Geometry: final body of the model. Coordinates: model frame, mm. Give positions to 0.01 mm unless a question says otherwise; leave off trailing zeros. Loops run counter-clockwise (first coordinate to the right, second up) from the corner with the lowest first, then second, coordinate; pieces in that order, holes last.
Autodesk Inventor part; units mm, degrees
ref_plane "YZ Plane" through (0, 0, 0) normal (1, 0, 0) x (0, 1, 0)
ref_plane "XZ Plane" through (0, 0, 0) normal (0, 1, 0) x (-1, 0, 0)
ref_plane "XY Plane" through (0, 0, 0) normal (0, 0, 1) x (1, 0, 0)
sketch "Sketch2" plane through (0, 0, 0) normal (1, 0, 0) x (0, 1, 0)
  line L0 (0, -180) -> (0, 0)
  line L1 (0, 0) -> (30, 0)
  line L2 (30, 0) -> (30, -3)
  line L3 (30, -3) -> (60, -3)
  line L4 (60, -3) -> (60, 0)
  line L5 (60, 0) -> (90, 0)
  line L6 (90, 0) -> (90, -3)
  line L7 (90, -3) -> (120, -3)
  line L8 (120, -3) -> (120, 0)
  line L9 (120, 0) -> (150, 0)
  line L10 (150, 0) -> (150, -3)
  line L11 (150, -3) -> (180, -3)
  line L12 (180, -3) -> (180, 0)
  line L13 (180, 0) -> (210, 0)
  line L14 (210, 0) -> (210, -3)
  line L15 (210, -3) -> (240, -3)
  line L16 (240, -3) -> (240, 0)
  line L17 (240, 0) -> (250, 0)
  line L18 (153.75, -180) -> (153.75, -80)
  line L19 (153.75, -80) -> (250, 0)
  line L20 (0, -90) -> (37, -90) construction
  line L21 (0, -180) -> (30, -180)
  line L22 (30, -180) -> (30, -177)
  line L23 (30, -177) -> (60, -177)
  line L24 (60, -177) -> (60, -180)
  line L25 (60, -180) -> (90, -180)
  line L26 (90, -180) -> (90, -177)
  line L27 (90, -177) -> (120, -177)
  line L28 (120, -177) -> (120, -180)
  line L29 (120, -180) -> (150, -180)
  line L30 (150, -180) -> (150, -177)
  line L31 (150, -177) -> (153.75, -177)
  line L32 (153.75, -180) -> (180, -180)
  line L33 (153.75, -180) -> (0, -180)
  point P0 (180, -177)
  point P1 (210, -180)
  dimension "d25" = 180
  dimension "d26" = 250
  dimension "d27" = 30
  dimension "d28" = 3
  dimension "d29" = 30
  dimension "d30" = 3
  dimension "d31" = 30
  dimension "d32" = 3
  dimension "d33" = 30
  dimension "d34" = 3
  dimension "d35" = 30
  dimension "d36" = 3
  dimension "d37" = 30
  dimension "d38" = 3
  dimension "d39" = 30
  dimension "d40" = 3
  dimension "d41" = 30
  dimension "d42" = 3
  dimension "d43" = 10
  dimension "d47" = 203
  dimension "d51" = 100
extrude "Extrusion2" add sketch "Sketch2" along normal blind 3 contours L0 L1 L2 L3 L4 L5 L6 L7 L8 L9 L10 L11 L12 L13 L14 L15 L16 L17 L19 L18 L31 L30 L29 L28 L27 L26 L25 L24 L23 L22 L21
properties part number "Q side 1" material "ABS Plastic"
Item 1: Section query C-C on z = -167.5. Return loops of the section in (x, y).
Values follow:
outline: (0, 0) - (3, 0) - (3, 153.75) - (0, 153.75) - close
Item 2: Pin query (flat end, axial travel): pin 1 (0.9 mm diameter, centred on x = 2, z = -178.5, fed in from -Y); pin 2 (1.5 mm diameter, centred on x = 1.5, z = -1, fed in from +Y); pin 3 (0.9 mm diameter, centred on x = 1.5, y = 171, fed in from +Z); pin 4 (0.9 mm diameter, centred on x = 1, y = 43.5, fed in from -Z). Return the tip coordinate at first contact, or that it passes through.
Values follow:
pin 1: stops at y = 0
pin 2: stops at y = 249.7
pin 3: stops at z = -3
pin 4: stops at z = -177
Item 3: Ray query, probe 1 along Y at (x, z) = (2.8, -139); probe 2 along Z at (x, y) = (2.05, 93); probe 3 along Z at (x, y) = (1.75, 157.5). Return the intervals inside material, ascending.
Values follow:
probe 1: y = 0 to 153.75
probe 2: z = -177 to -3
probe 3: z = -76.88 to -3
Item 4: Section query B-B on y = 50.5. Return loops of the section in (x, z), plus the area to 3 significant figures.
Values follow:
outline: (0, -177) - (3, -177) - (3, -3) - (0, -3) - close
area: 522 mm2
